Source: three-view drawing plus pictorial views. Frame: mm from the lowest corner of the part. A direction names the side the tool comes from. Give positions to 0.01 mm unless a question says otherwise; leave off trailing zeros. Loops run counter-clockwise (first coordinate to the right, second up) from the corner with the lowest first, then second, coordinate; pieces in that order, holes last. Notation, with made-up numbers: (-24, -0.75) - (-7, -0.75) arc R23 ccw to (-7, 8.25) - close; hole circle Ø7 at (47.5, 72). An arc over 180 degrees is marked (long way). Answer in a Markdown table with one row per item.
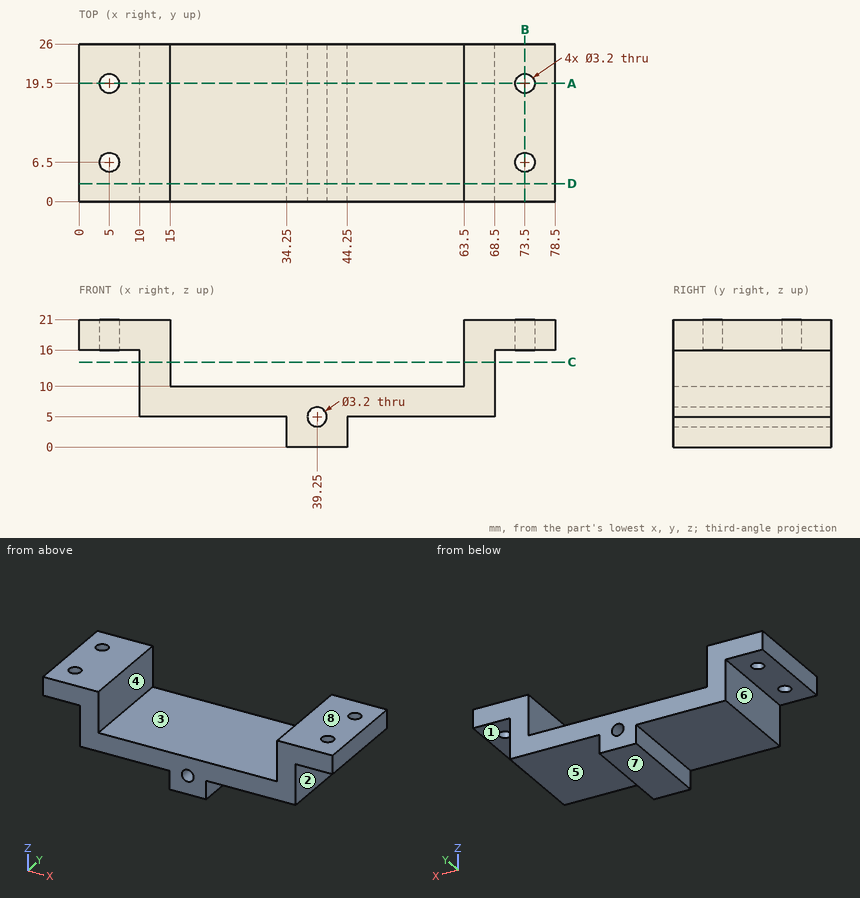
Q1. Cut plane C-C (z = 14). Output: boundary loops of the cut face in (x, y), and give its area (3 significant figures).
Check values:
| item | result |
|---|---|
| outline | (10, 0) - (15, 0) - (15, 26) - (10, 26) - close; (63.5, 0) - (68.5, 0) - (68.5, 26) - (63.5, 26) - close |
| area | 260 mm² |
Q2. Material intervals for line 1 along Y through (x, z) = (73.5, 17.9); line 2 along X through (y, z) = (17.75, 11); line 3 along Z through (x, y) = (64.5, 13.25), sorted ascending.
Check values:
| item | result |
|---|---|
| line 1 | 0 to 4.9, 8.1 to 17.9, 21.1 to 26 |
| line 2 | 10 to 15, 63.5 to 68.5 |
| line 3 | 5 to 21 |
Q3. Cut plane B-B (x = 73.5). Output: boundary loops of the cut face in (y, z).
Check values:
| item | result |
|---|---|
| outline | (0, 16) - (4.9, 16) - (4.9, 21) - (0, 21) - close; (8.1, 16) - (17.9, 16) - (17.9, 21) - (8.1, 21) - close; (21.1, 16) - (26, 16) - (26, 21) - (21.1, 21) - close |
Q4. First-contact query: pin 1 (3 mm diameter, centred on x = 66.5, y = 14.5, fed in from -Z); pin 2 (3.5 mm diameter, centred on y = 9, z = 15, fed in from -X); pin 3 (3 mm diameter, centred on x = 73, y = 14, fed in from -Z); pin 4 (3 mm diameter, centred on y = 17.5, z = 12, fed in from +X). Flat tips, straight axial feed; report the tip coordinate or a pass-through.
Check values:
| item | result |
|---|---|
| pin 1 | z = 5 |
| pin 2 | x = 0 |
| pin 3 | z = 16 |
| pin 4 | x = 68.5 |
Q5. Cut plane A-A (y = 19.5). Output: boundary loops of the cut face in (x, z).
Check values:
| item | result |
|---|---|
| outline | (0, 16) - (3.4, 16) - (3.4, 21) - (0, 21) - close; (6.6, 16) - (10, 16) - (10, 5) - (34.25, 5) - (34.25, 0) - (44.25, 0) - (44.25, 5) - (68.5, 5) - (68.5, 16) - (71.9, 16) - (71.9, 21) - (63.5, 21) - (63.5, 10) - (15, 10) - (15, 21) - (6.6, 21) - close; (75.1, 16) - (78.5, 16) - (78.5, 21) - (75.1, 21) - close; hole circle Ø3.2 at (39.25, 5) |
Q6. Cut plane D-D (y = 3). Output: boundary loops of the cut face in (x, z).
Check values:
| item | result |
|---|---|
| outline | (0, 16) - (10, 16) - (10, 5) - (34.25, 5) - (34.25, 0) - (44.25, 0) - (44.25, 5) - (68.5, 5) - (68.5, 16) - (78.5, 16) - (78.5, 21) - (63.5, 21) - (63.5, 10) - (15, 10) - (15, 21) - (0, 21) - close; hole circle Ø3.2 at (39.25, 5) |
Q7. Draft query along X for the marked faces 1, 2 and 3. Return one class per face: pulls with the +X half, pulls with the -X half, needs draft (parallel to the pull), parting line crosses it, or undercut.
Check values:
| item | result |
|---|---|
| face 1 | needs draft |
| face 2 | pulls with the +X half |
| face 3 | undercut |
Q8. Reachability of the marked faces 4, 5, 6, 7 and 8 from +Z, -Z, +X, -X, +Y, -Y: full face, straight path, thin tool, end or side. Return the list, or none.
Check values:
| item | result |
|---|---|
| face 4 | +Z, +Y, -Y |
| face 5 | -Z, +X, +Y, -Y |
| face 6 | -Z, -X, +Y, -Y |
| face 7 | -Z, +X, -X, +Y, -Y |
| face 8 | +Z, +X, -X, +Y, -Y |
